Solid Edge part; units mm, degrees
sketch "Sketch1" plane through (0, 0, 0) normal (0, -1, 0) x (1, 0, 0)
  line L0 (-12.1652, 21.9294) -> (17.8348, 1.9294)
  line L1 (17.8348, -28.0706) -> (17.8348, 1.9294)
  line L2 (-42.1652, -28.0706) -> (17.8348, -28.0706)
  line L3 (-42.1652, -28.0706) -> (-42.1652, 1.9294)
  line L4 (-12.1652, 21.9294) -> (-42.1652, 1.9294)
extrude "Protrusion1" add sketch "Sketch1" against normal blind 40
sketch "Sketch2" plane through (17.8348, 20, -13.0706) normal (1, 0, 0) x (0, 1, 0)
  line L0 (-10, -15) -> (-10, 5)
  line L1 (-10, 5) -> (10, 5)
  line L2 (10, 5) -> (10, -15)
  line L3 (10, -15) -> (-10, -15)
extrude "ExtrudedProtrusion_2" add sketch "Sketch2" along normal blind 40
Here's how the part is built. I have some questions about the finished solid (model axes, mm). A direction names the side the tool comes from. Round coordinates to 2 decimals unless told otherwise and drop trailing zeros. Loops run counter-clockwise (first coordinate to the right, second up) from the corner with the lowest first, then second, coordinate; pieces in that order, holes last.
1. Suppose I cut it at B-B, the plane z = -13. Please give me the cut outline in (x, y), and give its area (3 significant figures).
Answers:
outline: (-42.17, 0) - (17.83, 0) - (17.83, 10) - (57.83, 10) - (57.83, 30) - (17.83, 30) - (17.83, 40) - (-42.17, 40) - close
area: 3,200 mm2
2. Will these pins go through, and if not, where does the flat tip stop? pin 1 (1.5 mm diameter, centred on x = 28.5, z = -21, fed in from +Y); pin 2 (6 mm diameter, centred on x = 32, z = -14, fed in from -Y); pin 3 (4 mm diameter, centred on x = -24.5, y = 29, fed in from +Z).
Answers:
pin 1: stops at y = 30
pin 2: stops at y = 10
pin 3: stops at z = 15.04
3. Suppose I cut it at A-A, the plane y = 24. Please give me the cut outline in (x, z).
Answers:
outline: (-42.17, -28.07) - (57.83, -28.07) - (57.83, -8.07) - (17.83, -8.07) - (17.83, 1.93) - (-12.17, 21.93) - (-42.17, 1.93) - close
4. If I drill on probe 1 along X at (y, z) = (3.5, -0.5); probe 2 along Y at (x, z) = (37.5, -9); probe 3 along Z at (x, y) = (30, 18), over which ranges is the centre line in solid material (lowest first)?
Answers:
probe 1: x = -42.17 to 17.83
probe 2: y = 10 to 30
probe 3: z = -28.07 to -8.07
5. For faces 1 (the face through (38, 10, -18)), 2 (the face through (38, 30, -18)), 3 (the face through (38, 20, -8.071)), which set-ups out of +Z, -Z, +X, -X, +Y, -Y let a thin tool reach every point of the face, with its end or its side?
Answers:
face 1: +Z, -Z, +X, -Y
face 2: +Z, -Z, +X, +Y
face 3: +Z, +X, +Y, -Y
6. Suppose I cut it at C-C, the plane y = 5. Please give me the cut outline in (x, z), and give its area (3 significant figures).
Answers:
outline: (-42.17, -28.07) - (17.83, -28.07) - (17.83, 1.93) - (-12.17, 21.93) - (-42.17, 1.93) - close
area: 2,400 mm2
7. Suppose I cut it at D-D, the plane x = 19. Please give me the cut outline in (y, z), and give its area (3 significant figures).
Answers:
outline: (10, -28.07) - (30, -28.07) - (30, -8.07) - (10, -8.07) - close
area: 400 mm2
